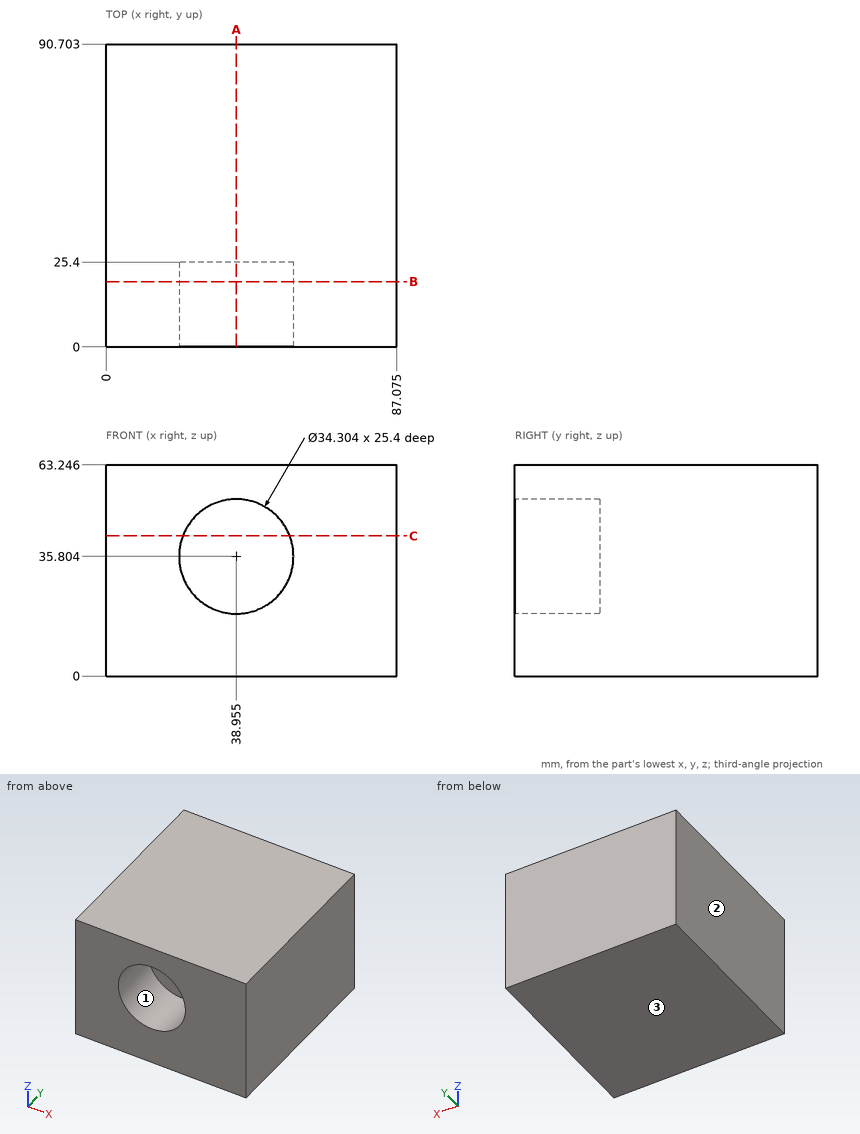
Here's the drawing with two shaded views (mm, measured from the low corner). I have some questions. Give positions to 0.01 mm unless a question says otherwise; leave off trailing zeros. Write each loop counter-clockwise with the first axis right and the second up, starting at its lowest first coordinate (ties: lowest second). Pieces come first, ordered by that corner, then holes. Notation, with made-up numbers: (-20.5, 77.25) -> (16.5, 77.25) arc R10 cw to (16.5, 92.25) -> close; hole circle Ø10 at (19, 21). An arc over 180 degrees is marked (long way). Use one line per item in the form item = value.
1) Suppose I cut it at A-A (x = 39). Please give me the cut outline in (y, z) (1 decimal).
Verdict:
outline = (0, 0) -> (90.7, 0) -> (90.7, 63.2) -> (0, 63.2) -> (0, 53) -> (25.4, 53) -> (25.4, 18.7) -> (0, 18.7) -> close
2) Suppose I cut it at B-B (y = 19.5). Please give me the cut outline in (x, z) (1 decimal).
Verdict:
outline = (0, 0) -> (87.1, 0) -> (87.1, 63.2) -> (0, 63.2) -> close; hole circle Ø34.3 at (39, 35.8)
3) Suppose I cut it at C-C (z = 42). Please give me the cut outline in (x, y) (1 decimal), and give its area (3 significant figures).
Verdict:
outline = (0, 0) -> (23, 0) -> (23, 25.4) -> (54.9, 25.4) -> (54.9, 0) -> (87.1, 0) -> (87.1, 90.7) -> (0, 90.7) -> close
area = 7,090 mm2
4) If I drill on L1, parallel to Y at x = 54, z = 39; L2, parallel to X at y = 4, z = 49.5 (1 decimal); L3, parallel to X at y = 13.5, z = 41 (1 decimal), over which ranges is the centre line in solid material (lowest first)? Write a range as [from, to].
Verdict:
L1 = [25.4, 90.7]
L2 = [0, 28.6], [49.3, 87.1]
L3 = [0, 22.6], [55.3, 87.1]
5) I'm going to push flat-ended pins straight in: pin 1 (8 mm diameter, centred on y = 27.5, z = 20, fed in from -X); pin 2 (17 mm diameter, centred on x = 41, z = 33, fed in from -Y). Where does each tip first touch, or does it pass through?
Verdict:
pin_1 = 0
pin_2 = 25.4
6) We'd pull the mould along X, two halves only. Please class the marked faces 1, 2 and 3: +X half, -X half, draft (parallel to the pull), parting line (faces both ways), or undercut.
Verdict:
face_1 = undercut
face_2 = -X half
face_3 = draft
